Read the model definition and answer for the solid it produces. Units are mm, in the model's axes. Face numbers are marked on the shaded views. A direction names the side the tool comes from. Coordinates: 2 decimals unless noted, no trailing zeros. Write each loop counter-clockwise with the first axis right and the second up, starting at its lowest first coordinate (ties: lowest second). Pieces come first, ordered by that corner, then holes.
(1) Section C-C on x = 11 is taken. Write down the section's boundary in (y, z).
(2) Section D-D on z = -36 is taken. Write down the section's boundary in (x, y).
(3) The mould has two halves that part along Y. Classify the marked faces 1, 2 and 3: +Y half, -Y half, draft (parallel to the pull), parting line (faces both ways), or undercut.
(4) Which of the six approach directions +Z, -Z, +X, -X, +Y, -Y give full straight-line access (tool end or side, diameter ignored) to the marked faces 4, 5 and 6?
(5) Section A-A on y = 23.56 is taken. Write down the section's boundary in (x, z).
(6) Find the intervals of material crossed by probe 1 along Z at (x, y) = (1, 24); probe 2 along Y at (x, z) = (21.3, -15) (1 decimal); probe 3 along Y at (x, z) = (21, -15) (1 decimal), in increasing order.
(7) Section B-B on z = -15 is taken. State how many separate pieces and enclosed holes the cut face has, then the cut area to 3 significant figures.
(8) Given pin 1 (6 mm diameter, centred on x = 12, y = 12, fed in from +Z); pin 2 (12 mm diameter, centred on x = 8.5, z = -34.5, fed in from -Y); pin 3 (15 mm diameter, centred on y = 6.56, z = -15, fed in from +X); pin 4 (6 mm diameter, centred on x = -8, z = -23.5, fed in from -Y), each flat-ended and moving along its own axis, determine where each tip first touches the part or whether it passes through.
Autodesk Inventor part; units mm, degrees
ref_plane "Work Plane1" through (0, 0, -15) normal (0, 0, 1) x (1, 0, 0)
ref_plane "YZ Plane" through (0, 0, 0) normal (1, 0, 0) x (0, 1, 0)
ref_plane "XZ Plane" through (0, 0, 0) normal (0, 1, 0) x (-1, 0, 0)
sketch "Sketch1" plane through (0, 0, 0) normal (0, 0, 1) x (1, 0, 0)
  line L0 (0, 0) -> (25, 0)
  line L1 (25, 0) -> (25, 40)
  line L2 (25, 40) -> (0, 40)
  line L3 (0, 40) -> (0, 0)
  dimension "d1" = 25
  dimension "d2" = 40
  dimension "d3" = 25
extrude "Extrusion1" add sketch "Sketch1" against normal blind 30
sketch "Sketch2" plane through (25, 0, 0) normal (1, 0, 0) x (0, 0, -1)
  line L0 (0, 0) -> (30, 0)
  circle A0 centre (15, 6.56) radius 2.46
extrude "Extrusion2" cut sketch "Sketch2" against normal blind 30
sketch "Sketch3" plane through (0, 0, 0) normal (-1, 0, 0) x (0, 0, 1)
  line L0 (0, 0) -> (-30, 0)
  line L1 (-25.05, 0) -> (-4.95, 0)
  line L2 (-4.95, 0) -> (-4.95, 33.12)
  line L3 (-4.95, 33.12) -> (-25.05, 33.12)
  line L4 (-25.05, 33.12) -> (-25.05, 0)
  dimension "d11" = 20.1
extrude "Extrusion3" cut sketch "Sketch3" against normal blind 20
sketch "Sketch4" plane through (0, 0, 0) normal (0, -1, 0) x (1, 0, 0)
  line L0 (20, -4.95) -> (20, -25.05)
  line L1 (20, -15) -> (25, -15)
  line L2 (25, 0) -> (25, -30)
  line L3 (20, -8.025) -> (25, -8.025)
  line L4 (25, -8.025) -> (25, -21.975)
  line L5 (25, -21.975) -> (20, -21.975)
  line L6 (20, -21.975) -> (20, -8.025)
  line L7 (20, -8.025) -> (25, -21.975) construction
  line L8 (25, -8.025) -> (20, -21.975) construction
  line L9 (25, -12.54) -> (25, -17.46)
  point P0 (0, 0)
  point P1 (22.5, -15)
  dimension "d14" = 13.95
extrude "Extrusion4" add sketch "Sketch4" along normal blind 15
sketch "Sketch5" plane through (20, 0, 0) normal (-1, 0, 0) x (0, 0, 1)
  circle A0 centre (-15, 6.56) radius 2.46
  circle A1 centre (-15, 6.56) radius 4.7025
  circle A2 centre (-15, 6.56) radius 2.46
  circle A3 centre (-15, 6.56) radius 2.46
  point P0 (0, 0)
  dimension "d17" = 9.405
extrude "Extrusion5" cut sketch "Sketch5" against normal blind 2.1
sketch "Sketch6" plane through (25, 0, 0) normal (1, 0, 0) x (0, 0, -1)
  circle A0 centre (15, 6.56) radius 4.7025
  line L0 (15, 6.56) -> (15, 23.56)
  circle A1 centre (15, 23.56) radius 2.46
  point P0 (0, 0)
  dimension "d20" = 17
  dimension "d21" = 4.92
extrude "Extrusion6" cut sketch "Sketch6" against normal blind 10 contours A1
sketch "Sketch7" plane through (20, 0, 0) normal (-1, 0, 0) x (0, 0, 1)
  circle A0 centre (-15, 23.56) radius 2.46
  circle A1 centre (-15, 23.56) radius 4.7025
  point P0 (0, 0)
  dimension "d24" = 9.405
extrude "Extrusion7" cut sketch "Sketch7" against normal blind 2.1
sketch "Sketch9" plane through (25, 0, 0) normal (1, 0, 0) x (0, 0, -1)
  circle A0 centre (15, 6.56) radius 2.46
  circle A1 centre (15, 6.56) radius 2.46
  circle A2 centre (15, 23.56) radius 2.46
  circle A3 centre (15, 23.56) radius 2.46
  line L0 (30, 40) -> (30, 0)
  line L1 (30, 0) -> (30, 40)
  line L2 (30, 40) -> (0, 40)
  line L3 (0, 40) -> (0, 0)
  line L4 (0, 0) -> (8.025, 0)
  line L5 (21.975, 0) -> (21.975, -15)
  line L6 (21.975, -15) -> (8.025, -15)
  line L7 (8.025, -15) -> (8.025, 0)
  line L8 (0, 0) -> (8.025, 0)
  line L9 (21.975, 0) -> (30, 0)
extrude "Extrusion8" add sketch "Sketch9" along normal blind 5
sketch "Sketch10" plane through (0, 40, 0) normal (0, 1, 0) x (1, 0, 0)
  line L0 (0, 30) -> (30, 30)
  line L1 (30, 0) -> (0, 0)
  line L2 (0, 30) -> (30, 30)
  line L3 (30, 30) -> (30, 0)
  line L4 (30, 0) -> (0, 0)
  line L5 (0, 0) -> (0, 30)
extrude "Extrusion9" add sketch "Sketch10" along normal blind 30
sketch "Sketch12" plane through (30, 0, 0) normal (1, 0, 0) x (0, 0, -1)
  circle A0 centre (15, 6.56) radius 2.46
  line L0 (15, 6.56) -> (15, 15.06)
  circle A1 centre (15, 15.06) radius 2.525
  point P0 (0, 0)
  dimension "d31" = 8.5
  dimension "d33" = 5.05
extrude "Extrusion10" cut sketch "Sketch12" against normal blind 30 contours A1
sketch "Sketch14" plane through (0, 0, 0) normal (0, 0, 1) x (1, 0, 0)
  line L0 (30, 70) -> (0, 70)
  line L1 (0, 70) -> (0, 85)
  line L2 (30, 0) -> (30, 70)
  line L3 (30, 100) -> (30, 70)
  line L4 (-12, 120) -> (15, 120)
  line L5 (-9.5, 118) -> (-7, 110)
  line L6 (-9.5, 118) -> (-12, 120)
  line L7 (-9.5, 102) -> (-7, 110)
  line L8 (-9.5, 102) -> (-12, 100)
  line L9 (30, 105) -> (15, 120)
  line L10 (30, 105) -> (30, 100)
  line L11 (0, 85) -> (0, 100)
  line L12 (0, 100) -> (-12, 100)
  point P0 (0, 0)
  dimension "d60" = 20
  dimension "d64" = 12
extrude "Extrusion12" add sketch "Sketch14" against normal blind 30
sketch "Sketch15" plane through (0, 0, -25.05) normal (-1, 0, 0) x (0, 0, 1)
  line L0 (0, 33.12) -> (20.1, 33.12)
  line L1 (20.1, 33.12) -> (20.1, 0)
  line L2 (0, 33.12) -> (20.1, 33.12)
  line L3 (20.1, 33.12) -> (20.1, 31.1)
  line L4 (20.1, 31.1) -> (0, 31.1)
  line L5 (0, 31.1) -> (0, 33.12)
  point P0 (25.05, 0)
  dimension "d57" = 2.02
extrude "Extrusion13" add sketch "Sketch15" against normal blind 20
sketch "Sketch20" plane through (0, 0, 0) normal (0, 0, 1) x (1, 0, 0)
  line L0 (0, 100) -> (-12, 100)
  line L1 (0, 100) -> (-12, 100)
  line L2 (-12, 100) -> (-9.5, 102)
  line L3 (-12, 100) -> (-9.5, 102)
  line L4 (-9.5, 102) -> (-7, 110)
  line L5 (-9.5, 102) -> (-7, 110)
  line L6 (-7, 110) -> (-9.5, 118)
  line L7 (-7, 110) -> (-9.5, 118)
  line L8 (-9.5, 118) -> (-12, 120)
  line L9 (-9.5, 118) -> (-12, 120)
  line L10 (-12, 120) -> (15, 120)
  line L11 (-12, 120) -> (15, 120)
  line L12 (15, 120) -> (30, 105)
  line L13 (15, 120) -> (30, 105)
  line L14 (30, 105) -> (30, 90)
  line L15 (30, 0) -> (30, 105)
  line L16 (30, 90) -> (0, 90)
  line L17 (0, 90) -> (0, 100)
  point P0 (0, 0)
  dimension "d65" = 15
  dimension "d66" = 30
extrude "Extrusion14" add sketch "Sketch20" along normal blind 15
ref_plane "Work Plane1" through (0, 0, -15) normal (0, 0, 1) x (1, 0, 0)
mirror "Mirror1" about plane through (0, 0, -15) normal (0, 0, 1) of "Extrusion14"
properties part number "rec_b_16mm_x_60mm"
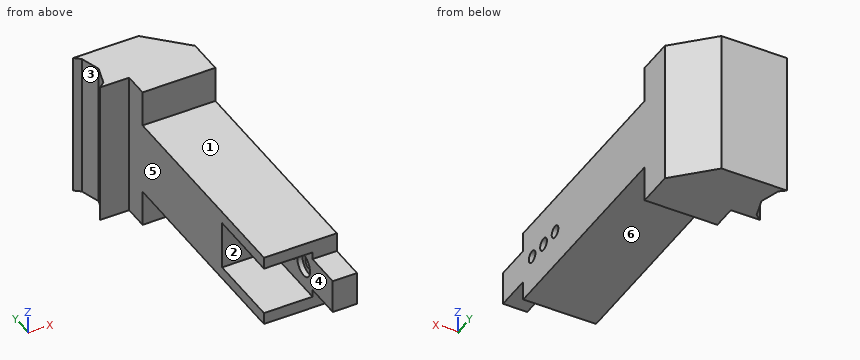
Response:
1. outline: (0, -30) - (90, -30) - (90, -45) - (120, -45) - (120, 15) - (90, 15) - (90, 0) - (0, 0) - (0, -4.95) - (31.1, -4.95) - (31.1, -25.05) - (0, -25.05) - close
2. outline: (-12, 100) - (0, 100) - (0, 90) - (30, 90) - (30, 105) - (15, 120) - (-12, 120) - (-9.5, 118) - (-7, 110) - (-9.5, 102) - close
3. face 1: draft
3. face 2: -Y half
3. face 3: undercut
4. face 4: -X, -Y
4. face 5: +Z, -Z, -X, -Y
4. face 6: -Z, +X, -X, -Y
5. outline: (0, -30) - (30, -30) - (30, -17.46) - (22.1, -17.46) - (22.1, -19.7) - (20, -19.7) - (20, -25.05) - (0, -25.05) - close; (0, -4.95) - (20, -4.95) - (20, -10.3) - (22.1, -10.3) - (22.1, -12.54) - (30, -12.54) - (30, 0) - (0, 0) - close
6. probe 1: z = -30 to -25.05, -4.95 to 0
6. probe 2: y = -15 to 1.9, 11.3 to 12.5, 17.6 to 18.9, 28.3 to 113.7
6. probe 3: y = -15 to 1.9, 11.3 to 12.5, 17.6 to 18.9, 28.3 to 114
7. separate pieces: 4
7. enclosed holes: 0
7. area: 3,020 mm2
8. pin 1: stops at z = 0
8. pin 2: stops at y = 0
8. pin 3: stops at x = 30
8. pin 4: stops at y = 100
